Input: part model. Units: mm. Frame: model coordinates. Round coordinates to 2 decimals unless told otherwise and drop trailing zeros. Loops run counter-clockwise (first coordinate to the right, second up) from the corner with the lowest first, then second, coordinate; pieces in that order, holes last. Notation, with made-up numbers: M 40.25,31.25 L 50.25,31.25 A30 cw 50.25,65.25 Z; hole C -26,-29.5 d9. An arc over 180 degrees is marked long. Return JSON: item names as keys, results as strings. Group by question number.
1) Section A-A (x = 0). Output: boundary loops of the cut face in (y, z), plus the area to 3 significant figures.
2) Material intervals for line 1 (Y direction, x = 0, z = 6); line 2 (X direction, y = -1.5, z = 4); line 3 (X direction, y = 0.5, z = 2), sorted ascending. Write a range as from..to.
3) Contact query for flat-ended pins moving along their axis: P1, Ø2, axis at x = 3.5, z = 8.5, coming from the -Y side; P2, Ø2, axis at x = 1, y = 1, coming from the +Z side; P3, Ø1.5, axis at y = -4.5, z = 7.5, coming from the -X side. Output: stop coordinate, or through.
4) Section C-C (z = 4.75). Output: boundary loops of the cut face in (x, y), plus the area to 3 significant figures.
5) Section D-D (y = 6). Output: boundary loops of the cut face in (x, z), plus the area to 3 significant figures.
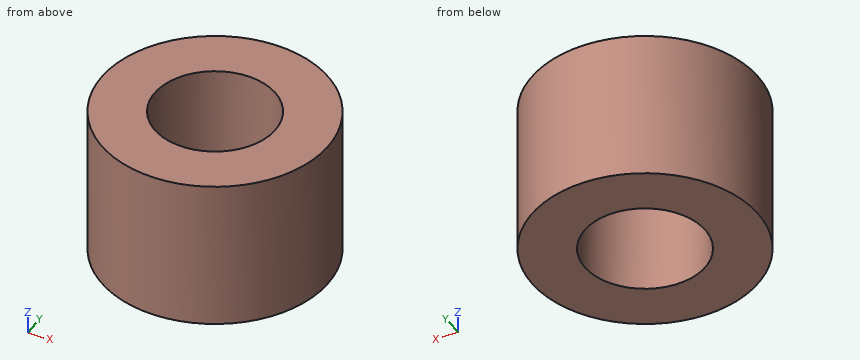
from build123d import *

# Parameters (mm, degrees)
F0_R     = 7.5
F0_R_2   = 4
F1_DEPTH = 10
F2_W     = 30
F2_H     = 1


with BuildPart() as f1:
    # F0 (on Top) → F1 (new body)
    with BuildSketch(Plane.XY):
        Circle(F0_R)
        Circle(F0_R_2, mode=Mode.SUBTRACT)
    extrude(amount=F1_DEPTH)


with BuildPart() as f3:
    # F2 (on Front) → F3 (revolve)
    with BuildSketch(Plane.XZ):
        with Locations((31.168116, 42.156867)):
            Rectangle(F2_W, F2_H)
    revolve(axis=Axis((31.168116, 0, 42.656867), (1, 0, 0)))


solid = f1.part
Returned:
{
 "1": {"outline": "M -7.5,0 L -4,0 L -4,10 L -7.5,10 Z; M 4,0 L 7.5,0 L 7.5,10 L 4,10 Z", "area": "70.0 mm^2"},
 "2": {"line 1": "y = -7.5..-4, 4..7.5", "line 2": "x = -7.35..-3.71, 3.71..7.35", "line 3": "x = -7.48..-3.97, 3.97..7.48"},
 "3": {"P1": "stops at y = -7.07", "P2": "passes through", "P3": "stops at x = -6.5"},
 "4": {"outline": "C 0,0 d15; hole C 0,0 d8", "area": "126 mm^2"},
 "5": {"outline": "M -4.5,0 L 4.5,0 L 4.5,10 L -4.5,10 Z", "area": "90.0 mm^2"}
}
